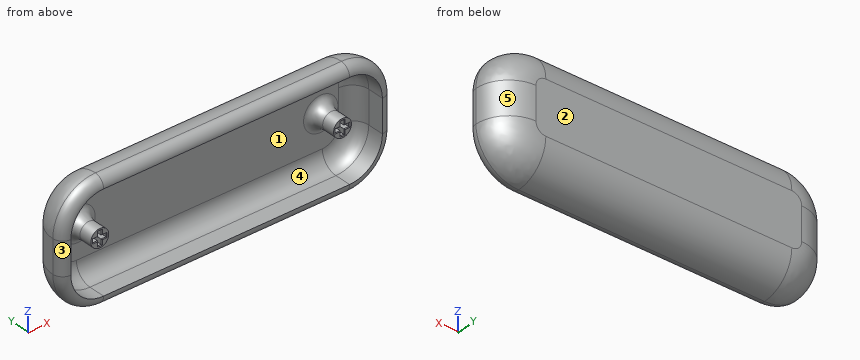
```python
from build123d import *

# Parameters (mm, degrees)
EXTRUDE_1_DEPTH  = 10
SHELL_2_T        = 3
FILLET_3_R       = 10
FILLET_4_R       = 3
SKETCH_2_R       = 2.725
EXTRUDE_2_DEPTH  = 8
FILLET_7_R       = 5
CHAMFER_1_SIZE   = 0.2
CHAMFER_2_SIZE   = 0.2
FILLET_9_SIZE    = 2.5
FILLET_9_SIZE_2  = 4
FILLET_10_SIZE   = 2.5
FILLET_10_SIZE_2 = 4


# Some blends are built 0.0001 mm under size
with BuildPart() as part:
    # 草图1 → 凸台-拉伸1 (new body)
    with BuildSketch(Plane(origin=(0, 0, 0), x_dir=(1, 0, 0), z_dir=(0, 1, 0))):
        with BuildLine():
            Line((-37.5, 15), (37.5, 15))
            ThreePointArc((37.5, 15), (44.571067812, 12.071067812), (47.5, 5))
            Line((47.5, 5), (47.5, -5))
            ThreePointArc((47.5, -5), (44.571067812, -12.071067812), (37.5, -15))
            Line((37.5, -15), (-37.5, -15))
            ThreePointArc((-37.5, -15), (-44.571067812, -12.071067812), (-47.5, -5))
            Line((-47.5, -5), (-47.5, 5))
            ThreePointArc((-47.5, 5), (-44.571067812, 12.071067812), (-37.5, 15))
        make_face()
    extrude(amount=EXTRUDE_1_DEPTH)

    # 抽壳2
    shell_2_openings = [part.faces().sort_by_distance(p)[0] for p in [
        (0, 0, 0),
    ]]
    offset(amount=SHELL_2_T, openings=shell_2_openings, kind=Kind.INTERSECTION)

    # 圆角3
    # the kernel refuses this fillet: 10 mm, written as the material it takes off along each edge
    with BuildSketch(Plane(origin=(37.5, 13, 5), x_dir=(1, 0, 0), z_dir=(0, 0, -1))) as fillet_3_piece_1:
        with BuildLine():
            CenterArc((13 - FILLET_3_R, FILLET_3_R), FILLET_3_R, 270, 90)
            Line((13 - FILLET_3_R, 0), (13, 0))
            Line((13, 0), (13, FILLET_3_R))
        make_face()
    revolve(axis=Axis((37.5, 13, 5), (0, -1, 0)), revolution_arc=90, mode=Mode.SUBTRACT)
    with BuildSketch(Plane(origin=(50.5, 13, 5), x_dir=(0, -1, 0), z_dir=(0, 0, -1)), Plane(origin=(-50.5, 13, -5), x_dir=(0, -1, 0), z_dir=(0, 0, 1))) as fillet_3_piece_2:
        with BuildLine():
            CenterArc((FILLET_3_R, FILLET_3_R), FILLET_3_R, 180, 90)
            Line((0, FILLET_3_R), (0, 0))
            Line((0, 0), (FILLET_3_R, 0))
        make_face()
    extrude(amount=10, mode=Mode.SUBTRACT)
    with BuildSketch(Plane(origin=(37.5, 13, -5), x_dir=(0, 0, -1), z_dir=(-1, 0, 0))) as fillet_3_piece_3:
        with BuildLine():
            CenterArc((13 - FILLET_3_R, FILLET_3_R), FILLET_3_R, 270, 90)
            Line((13 - FILLET_3_R, 0), (13, 0))
            Line((13, 0), (13, FILLET_3_R))
        make_face()
    revolve(axis=Axis((37.5, 13, -5), (0, -1, 0)), revolution_arc=90, mode=Mode.SUBTRACT)
    with BuildSketch(Plane(origin=(37.5, 13, -18), x_dir=(0, -1, 0), z_dir=(-1, 0, 0)), Plane(origin=(-37.5, 13, 18), x_dir=(0, -1, 0), z_dir=(1, 0, 0))) as fillet_3_piece_4:
        with BuildLine():
            CenterArc((FILLET_3_R, FILLET_3_R), FILLET_3_R, 180, 90)
            Line((0, FILLET_3_R), (0, 0))
            Line((0, 0), (FILLET_3_R, 0))
        make_face()
    extrude(amount=75, mode=Mode.SUBTRACT)
    with BuildSketch(Plane(origin=(-37.5, 13, -5), x_dir=(-1, 0, 0), z_dir=(0, 0, 1))) as fillet_3_piece_5:
        with BuildLine():
            CenterArc((13 - FILLET_3_R, FILLET_3_R), FILLET_3_R, 270, 90)
            Line((13 - FILLET_3_R, 0), (13, 0))
            Line((13, 0), (13, FILLET_3_R))
        make_face()
    revolve(axis=Axis((-37.5, 13, -5), (0, -1, 0)), revolution_arc=90, mode=Mode.SUBTRACT)
    with BuildSketch(Plane(origin=(-37.5, 13, 5), x_dir=(0, 0, 1), z_dir=(1, 0, 0))) as fillet_3_piece_6:
        with BuildLine():
            CenterArc((13 - FILLET_3_R, FILLET_3_R), FILLET_3_R, 270, 90)
            Line((13 - FILLET_3_R, 0), (13, 0))
            Line((13, 0), (13, FILLET_3_R))
        make_face()
    revolve(axis=Axis((-37.5, 13, 5), (0, -1, 0)), revolution_arc=90, mode=Mode.SUBTRACT)

    # 圆角4
    fillet_4_edges = [part.edges().sort_by_distance(p)[0] for p in [
        (50.5, 0, 0),
        (46.692388155, 0, 14.192388155),
        (0, 0, 18),
        (-46.692388155, 0, 14.192388155),
        (-50.5, 0, 0),
        (-46.692388155, 0, -14.192388155),
        (0, 0, -18),
        (46.692388155, 0, -14.192388155),
    ]]
    fillet(fillet_4_edges, radius=FILLET_4_R - 0.0001)  # a hair under: the kernel refuses the full size

    # 草图2 → 凸台-拉伸2 (add)
    # profile 1 of 2: a face of its own
    with BuildSketch(Plane(origin=(0, 10, 0), x_dir=(-1, 0, 0), z_dir=(0, -1, 0))):
        with Locations(Location((37, 0, 0), (0, 0, 270))):
            Circle(SKETCH_2_R)
        Polygon((34.95, -0.55), (34.95, 0.55), (36.45, 0.55), (36.45, 2.05), (37.55, 2.05), (37.55, 0.55), (39.05, 0.55), (39.05, -0.55), (37.55, -0.55), (37.55, -2.05), (36.45, -2.05), (36.45, -0.55), align=None, mode=Mode.SUBTRACT)
    # profile 2 of 2: a face of its own
    with BuildSketch(Plane(origin=(0, 10, 0), x_dir=(-1, 0, 0), z_dir=(0, -1, 0))):
        with Locations(Location((-37, 0, 0), (0, 0, 90))):
            Circle(SKETCH_2_R)
        Polygon((-37.55, 0.55), (-37.55, 2.05), (-36.45, 2.05), (-36.45, 0.55), (-34.95, 0.55), (-34.95, -0.55), (-36.45, -0.55), (-36.45, -2.05), (-37.55, -2.05), (-37.55, -0.55), (-39.05, -0.55), (-39.05, 0.55), align=None, mode=Mode.SUBTRACT)
    extrude(amount=EXTRUDE_2_DEPTH)

    # 圆角7
    fillet_7_edges = [part.edges().sort_by_distance(p)[0] for p in [
        (-44.571067812, 10, 12.071067812),
        (0, 10, 15),
        (44.571067812, 10, 12.071067812),
        (47.5, 10, 0),
        (44.571067812, 10, -12.071067812),
        (0, 10, -15),
        (-44.571067812, 10, -12.071067812),
        (-47.5, 10, 0),
    ]]
    fillet(fillet_7_edges, radius=FILLET_7_R)

    # 倒角1
    chamfer_1_edges = [part.edges().sort_by_distance(p)[0] for p in [
        (35.7, 2, -0.55),
        (37.55, 2, 1.3),
        (39.05, 2, 0),
        (38.3, 2, -0.55),
        (37.55, 2, -1.3),
        (37, 2, -2.05),
        (34.95, 2, 0),
        (35.7, 2, 0.55),
        (36.45, 2, 1.3),
        (37, 2, 2.05),
        (38.3, 2, 0.55),
        (36.45, 2, -1.3),
    ]]
    chamfer(chamfer_1_edges, length=CHAMFER_1_SIZE)

    # 倒角2
    chamfer_2_edges = [part.edges().sort_by_distance(p)[0] for p in [
        (-37, 2, -2.05),
        (-37.55, 2, -1.3),
        (-38.3, 2, -0.55),
        (-39.05, 2, 0),
        (-37.55, 2, 1.3),
        (-35.7, 2, -0.55),
        (-38.3, 2, 0.55),
        (-37, 2, 2.05),
        (-36.45, 2, 1.3),
        (-35.7, 2, 0.55),
        (-34.95, 2, 0),
        (-36.45, 2, -1.3),
    ]]
    chamfer(chamfer_2_edges, length=CHAMFER_2_SIZE)

    # 圆角9
    # an asymmetric fillet: 4, 2.5 mm, written as the material it adds along each edge
    with BuildSketch(Plane(origin=(37, 10, 0), x_dir=(0, 0, -1), z_dir=(-1, 0, 0))) as fillet_9_piece_1:
        with BuildLine():
            Bezier((2.725 + FILLET_9_SIZE, 0), (2.725, 0), (2.725, FILLET_9_SIZE_2), weights=[1, 0.707106781, 1])
            Line((2.725, FILLET_9_SIZE_2), (2.725, 0))
            Line((2.725, 0), (2.725 + FILLET_9_SIZE, 0))
        make_face()
    revolve(axis=Axis((37, 10, 0), (0, -1, 0)))

    # 圆角10
    # an asymmetric fillet: 4, 2.5 mm, written as the material it adds along each edge
    with BuildSketch(Plane(origin=(-37, 10, 0), x_dir=(0, 0, 1), z_dir=(1, 0, 0))) as fillet_10_piece_1:
        with BuildLine():
            Bezier((2.725 + FILLET_10_SIZE, 0), (2.725, 0), (2.725, FILLET_10_SIZE_2), weights=[1, 0.707106781, 1])
            Line((2.725, FILLET_10_SIZE_2), (2.725, 0))
            Line((2.725, 0), (2.725 + FILLET_10_SIZE, 0))
        make_face()
    revolve(axis=Axis((-37, 10, 0), (0, -1, 0)))


solid = part.part
```
Geometry: final body of the model. Coordinates: model frame, mm. Face numbers are marked on the shaded views. A direction names the side the tool comes from. Round coordinates to 2 decimals unless told otherwise and drop trailing zeros.
Item 1: Reachability of the marked faces 4 and 5 from +Z, -Z, +X, -X, +Y, -Y: full face, straight path, thin tool, end or side. Return the list, or none.
Checked values:
face 4: -Y
face 5: +Z, -Z, +X, +Y
Item 2: Mould query, pull axis X, two halves, no side actions, for the marked faces 1, 2 and 3. Classes: released by +X, released by -X, zero draft, split by the parting line, or undercut.
Checked values:
face 1: undercut
face 2: zero draft
face 3: released by -X
Item 3: Contact query for flat-ended pins moving along their axis: P1, Ø1.5, axis at x = -24.5, z = 0, coming from the -Y side; P2, Ø0.7, axis at y = 8, z = -1.5, coming from the +X side; P3, Ø1.2, axis at y = 7.5, z = 0, coming from the +X side; P4, Ø1, axis at y = 3.5, z = -5, coming from the -X side. Output: stop coordinate, or through.
Checked values:
P1: stops at y = 10
P2: stops at x = 49.35
P3: stops at x = 49.71
P4: stops at x = -50.5
Item 4: Section B-B, the plane y = 7.5. State how many separate pieces and enclosed holes the cut face has, plus the area to 3 significant figures.
Checked values:
separate pieces: 3
enclosed holes: 3
area: 653 mm2
Item 5: Line query: L1, parallel to X at y = 3.25, z = 5; L2, parallel to Z at x = -9, y = 3.25; L3, parallel to X at y = 6.5, z = 2.5. Output: solid intervals per line, ascending.
Checked values:
L1: x = -50.5 to -47.5, 47.5 to 50.5
L2: z = -18 to -15, 15 to 18
L3: x = -49.87 to -47.27, -38.13 to -35.87, 35.87 to 38.13, 47.27 to 49.87
